Work out the finished part from the listing and answer in its coordinate system (mm). A direction names the side the tool comes from. Coordinates: 2 decimals unless noted, no trailing zeros. Order: outer loops, then holes, each group sorted by start corner. A loop starts at its lowest first (then second) coordinate and runs counter-clockwise, first axis right, second up. Notation, with made-up numbers: (-10, 57) - (-2, 57) arc R17 cw to (-2, 81) - close; hole circle Ø4 at (81.25, -38.75). An arc over 180 degrees is marked (long way). Answer as a JSON object with one key per item and string values. Group by question number.
1) Section D-D (x = 4) is taken. Give the vertices of the cut face in (y, z) (3 decimals), plus the area to 3 significant figures.
2) Section A-A (y = 12.5) is taken. Give the vertices of the cut face in (x, z) (3 decimals).
3) Find the intervals of material crossed by line 1 along X through (y, z) = (37.75, -12.5) (3 decimals); line 2 along Y through (x, z) = (53.5, -12.5); line 3 along Z through (x, y) = (4, 6) (3 decimals), in increasing order.
4) Each of these flat-tipped pins is pushed along its axis until it touches: P1, Ø4, axis at x = 23, y = 27.5, coming from the +Z side; P2, Ø1.4, axis at y = 40.5, z = 2, coming from the -X side; P3, Ø1.5, axis at x = 21.5, z = 0, coming from the -Y side. Where does it stop, or does it pass through?
5) Section C-C (y = 37.5) is taken. Give the vertices of the cut face in (x, z) (3 decimals), plus the area to 3 significant figures.
6) Section B-B (z = -12.5) is taken. Give the vertices of the cut face in (x, y) (3 decimals).
7) The mould has two halves that part along Y. Classify faces 1 (the face through (25, 0, -12)), 2 (the face through (38, 36, -6.5)), 3 (the face through (8, 14.167, -13)): released by +Y, released by -Y, zero draft, split by the parting line, or undercut.
8) A tool of negligible diameter and unlimited length cuts with its end or side. For faces 4 (the face through (4, 37, -20)), 5 (the face through (-4.5, 36.6, -12.4)), 6 (the face through (35.22, 20.773, -23.274)), 7 (the face through (0, 41, -27)), from which of +Z, -Z, +X, -X, +Y, -Y can it reach the whole face along a straight path? Write none if from no direction.
from build123d import *

# Parameters (mm, degrees)
BOSS_EXTRUDE1_DEPTH = 55.5
CHAMFER1_SIZE       = 2
SKETCH4_W           = 8
SKETCH4_H           = 32.8
BOSS_EXTRUDE2_DEPTH = 5
SKETCH7_W           = 3.5
SKETCH7_H           = 6
CUT_EXTRUDE5_DEPTH  = 10
SKETCH5_R           = 3.375
CUT_EXTRUDE3_DEPTH  = 77.250596562
SKETCH6_R           = 3.375
CUT_EXTRUDE4_DEPTH  = 7.62
SKETCH8_W           = 9
SKETCH8_H           = 5
CUT_EXTRUDE6_DEPTH  = 9.167
BOSS_EXTRUDE3_DEPTH = 14.167
BOSS_EXTRUDE4_START = -29.407
BOSS_EXTRUDE4_DEPTH = 14.167
FILLET1_R           = 10
SKETCH10_W          = 15
SKETCH10_H          = 25
CUT_EXTRUDE7_DEPTH  = 20
SKETCH11_R          = 0.8
CUT_EXTRUDE8_DEPTH  = 8
SKETCH12_W          = 5
SKETCH12_H          = 12
CUT_EXTRUDE9_DEPTH  = 14.437


with BuildPart() as part:
    # Sketch1 → Boss-Extrude1 (new body)
    with BuildSketch(Plane(origin=(0, 0, 0), x_dir=(0, 0, -1), z_dir=(1, 0, 0))):
        Polygon((0, 0), (25, 0), (25, 19.787), (21.5, 21.787), (25, 23.787), (25, 43.574), (0, 43.574), (0, 23.787), (3.5, 21.787), (0, 19.787), align=None)
    extrude(amount=BOSS_EXTRUDE1_DEPTH)

    # Chamfer1
    chamfer1_edges = [part.edges().sort_by_distance(p)[0] for p in [
        (27.75, 43.574, 0),
        (27.75, 43.574, -25),
        (27.75, 0, -25),
        (27.75, 0, 0),
    ]]
    chamfer(chamfer1_edges, length=CHAMFER1_SIZE)

    # Sketch4 → Boss-Extrude2 (add)
    with BuildSketch(Plane(origin=(0, 43.574, 0), x_dir=(1, 0, 0), z_dir=(0, 1, 0))):
        with Locations((4, 12.5)):
            Rectangle(SKETCH4_W, SKETCH4_H)
    extrude(amount=-BOSS_EXTRUDE2_DEPTH)

    # Sketch7 → Cut-Extrude5 (cut)
    with BuildSketch(Plane(origin=(0, 43.574, 0), x_dir=(1, 0, 0), z_dir=(0, 1, 0))):
        with Locations((7.25, 2)):
            Rectangle(SKETCH7_W, SKETCH7_H)
        with Locations((7.25, 23)):
            Rectangle(SKETCH7_W, SKETCH7_H)
        with Locations((0.75, 2)):
            Rectangle(SKETCH7_W, SKETCH7_H)
        with Locations((0.75, 23)):
            Rectangle(SKETCH7_W, SKETCH7_H)
    extrude(amount=-CUT_EXTRUDE5_DEPTH, mode=Mode.SUBTRACT)

    # Sketch5 → Cut-Extrude3 (cut, through all)
    with BuildSketch(Plane(origin=(0, 43.574, 0), x_dir=(1, 0, 0), z_dir=(0, 1, 0))):
        with Locations(Location((4, 12.5, 0), (0, 0, 270))):
            Circle(SKETCH5_R)
    extrude(amount=-CUT_EXTRUDE3_DEPTH, mode=Mode.SUBTRACT)

    # Sketch6 → Cut-Extrude4 (cut, symmetric)
    with BuildSketch(Plane(origin=(0, 21.787, 0), x_dir=(-1, 0, 0), z_dir=(0, -1, 0))):
        Polygon((-4, 30), (4.5, 30), (4.5, -5), (-4, -5), (-15.5, -5), (-15.5, 30), align=None)
        with Locations(Location((-4, 12.5, 0), (0, 0, 270))):
            Circle(SKETCH6_R, mode=Mode.SUBTRACT)
    extrude(amount=CUT_EXTRUDE4_DEPTH, both=True, mode=Mode.SUBTRACT)

    # Sketch8 → Cut-Extrude6 (cut)
    with BuildSketch(Plane.XZ.offset(-29.407)):
        with Locations((4.5, -22.5)):
            Rectangle(SKETCH8_W, SKETCH8_H)
        with Locations((4.5, -2.5)):
            Rectangle(SKETCH8_W, SKETCH8_H)
    extrude(amount=-CUT_EXTRUDE6_DEPTH, mode=Mode.SUBTRACT)

    # Sketch9 → Boss-Extrude3 (add)
    with BuildSketch(Plane(origin=(0, 43.574, 0), x_dir=(1, 0, 0), z_dir=(0, 1, 0))):
        with BuildLine():
            Line((0, 20), (0, 5))
            ThreePointArc((0, 5), (-4.5, 12.5), (0, 20))
        make_face()
    extrude(amount=-BOSS_EXTRUDE3_DEPTH)

    # Sketch9<2> → Boss-Extrude4 (add)
    with BuildSketch(Plane(origin=(0, 43.574, 0), x_dir=(1, 0, 0), z_dir=(0, 1, 0)).offset(BOSS_EXTRUDE4_START)):
        with BuildLine():
            Line((0, 20), (0, 5))
            ThreePointArc((0, 5), (-4.5, 12.5), (0, 20))
        make_face()
    extrude(amount=-BOSS_EXTRUDE4_DEPTH)

    # Fillet1
    fillet1_edges = [part.edges().sort_by_distance(p)[0] for p in [
        (0, 7.0835, -20),
        (0, 7.0835, -5),
    ]]
    fillet(fillet1_edges, radius=FILLET1_R)

    # Sketch10 → Cut-Extrude7 (cut)
    with BuildSketch(Plane(origin=(55.5, 0, 0), x_dir=(0, 0, -1), z_dir=(1, 0, 0))):
        with Locations((12.5, 16.637)):
            Rectangle(SKETCH10_W, SKETCH10_H)
    extrude(amount=-CUT_EXTRUDE7_DEPTH, mode=Mode.SUBTRACT)

    # Sketch11 → Cut-Extrude8 (cut)
    with BuildSketch(Plane(origin=(55.5, 0, 0), x_dir=(0, 0, -1), z_dir=(1, 0, 0))):
        with Locations((12.5, 30.537)):
            Circle(SKETCH11_R)
    extrude(amount=-CUT_EXTRUDE8_DEPTH, mode=Mode.SUBTRACT)

    # Sketch12 → Cut-Extrude9 (cut)
    with BuildSketch(Plane(origin=(0, 43.574, 0), x_dir=(1, 0, 0), z_dir=(0, 1, 0))):
        with Locations((38, 12.5)):
            Rectangle(SKETCH12_W, SKETCH12_H)
    extrude(amount=-CUT_EXTRUDE9_DEPTH, mode=Mode.SUBTRACT)


solid = part.part
Report:
{
 "1": {"outline": "(0, -23) - (2, -25) - (14.167, -25) - (14.167, -15.875) - (0, -15.875) - close; (0, -9.125) - (14.167, -9.125) - (14.167, 0) - (2, 0) - (0, -2) - close; (29.407, -20) - (38.574, -20) - (38.574, -28.9) - (43.574, -28.9) - (43.574, -15.875) - (29.407, -15.875) - close; (29.407, -9.125) - (43.574, -9.125) - (43.574, 3.9) - (38.574, 3.9) - (38.574, -5) - (29.407, -5) - close", "area": "460 mm²"},
 "2": {"outline": "(-2.432, -18.056) arc R10 cw to (0, -24.593) - (0, -25) - (55.5, -25) - (55.5, -20) - (35.5, -20) - (35.5, -5) - (55.5, -5) - (55.5, 0) - (0, 0) - (0, -0.407) arc R10 cw to (-2.432, -6.944) arc R8.5 ccw to start; hole circle Ø6.75 at (4, -12.5)"},
 "3": {"line 1": "x = -4.5 to 0.625, 7.375 to 35.5, 40.5 to 55.5", "line 2": "y = 0 to 4.14, 29.14 to 29.74, 31.34 to 43.57", "line 3": "z = -25 to -15.875, -9.125 to 0"},
 "4": {"P1": "stops at z = 0", "P2": "stops at x = 0", "P3": "stops at y = 1.25"},
 "5": {"outline": "(0, -20) - (9, -20) - (9, -25) - (55.5, -25) - (55.5, 0) - (9, 0) - (9, -5) - (0, -5) arc R8.5 ccw to start; hole circle Ø6.75 at (4, -12.5); hole (35.5, -18.5) - (40.5, -18.5) - (40.5, -6.5) - (35.5, -6.5) - close", "area": "1,250 mm²"},
 "6": {"outline": "(-4.5, 0) - (0.625, 0) - (0.625, 14.167) - (-4.5, 14.167) - close; (-4.5, 29.407) - (0.625, 29.407) - (0.625, 43.574) - (-4.5, 43.574) - close; (7.375, 0) - (55.5, 0) - (55.5, 4.137) - (35.5, 4.137) - (35.5, 43.574) - (7.375, 43.574) - (7.375, 29.407) - (15.5, 29.407) - (15.5, 14.167) - (7.375, 14.167) - close; (40.5, 29.137) - (55.5, 29.137) - (55.5, 29.737) - (47.5, 29.737) - (47.5, 31.337) - (55.5, 31.337) - (55.5, 43.574) - (40.5, 43.574) - close"},
 "7": {"face 1": "released by -Y", "face 2": "zero draft", "face 3": "undercut"},
 "8": {"face 4": "none", "face 5": "-X, +Y", "face 6": "-Z, +X, -X", "face 7": "-Z, -X, +Y, -Y"}
}
